```python
from build123d import *

# Parameters (mm, degrees)
SKETCH1_W                                    = 60
SKETCH1_H                                    = 60
BOSS_EXTRUDE1_DEPTH                          = 3
SKETCH2_R                                    = 10.25
CUT_EXTRUDE1_DEPTH                           = 43.532340636
SKETCH3_R                                    = 1.45
SERVO_Y_MOUNT_D2P9_DEPTH                     = 3.01
SKETCH4_R                                    = 1.45
CUT_EXTRUDE5_DEPTH                           = 43.532340636
SKETCH5_R                                    = 1.2
GUIDERAIL1_D2P4_DEPTH                        = 3.01
SKETCH6_R                                    = 1.2
GUIDEBLOCK2_D2P4_DEPTH                       = 3.01
SKETCH7_R                                    = 2.1
GUIDEBLOCK2_HEADCOUNTERBORE_D4P2_DEPTH       = 2.05
SKETCH8_R                                    = 1.7
BENCH_XDROP_M3_CLEARANCE_HOLES_2X_D3P4_DEPTH = 3.5


with BuildPart() as part:
    # Sketch1 → Boss-Extrude1 (new body)
    with BuildSketch(Plane.XY):
        Rectangle(SKETCH1_W, SKETCH1_H)
    extrude(amount=BOSS_EXTRUDE1_DEPTH)

    # Sketch2 → Cut-Extrude1 (cut, through all)
    with BuildSketch(Plane.XY.offset(3)):
        Circle(SKETCH2_R)
    extrude(amount=-CUT_EXTRUDE1_DEPTH, mode=Mode.SUBTRACT)

    # Sketch3 → Servo_Y_Mount_D2p9 (cut)
    with BuildSketch(Plane(origin=(0, 0, 0), x_dir=(-1, 0, 0), z_dir=(0, 0, -1))):
        with Locations((18, -25)):
            Circle(SKETCH3_R)
        with Locations((25, -25)):
            Circle(SKETCH3_R)
    extrude(amount=-SERVO_Y_MOUNT_D2P9_DEPTH, mode=Mode.SUBTRACT)

    # Sketch4 → Cut-Extrude5 (cut, through all)
    with BuildSketch(Plane(origin=(0, 0, 0), x_dir=(-1, 0, 0), z_dir=(0, 0, -1))):
        with Locations((17, 27)):
            Circle(SKETCH4_R)
        with Locations((23, 27)):
            Circle(SKETCH4_R)
    extrude(amount=-CUT_EXTRUDE5_DEPTH, mode=Mode.SUBTRACT)

    # Sketch5 → GuideRail1_D2p4 (cut)
    with BuildSketch(Plane.XY.offset(3)):
        with Locations((-24, -15)):
            Circle(SKETCH5_R)
        with Locations((-24, 0)):
            Circle(SKETCH5_R)
        with Locations((-24, 15)):
            Circle(SKETCH5_R)
    extrude(amount=-GUIDERAIL1_D2P4_DEPTH, mode=Mode.SUBTRACT)

    # Sketch6 → GuideBlock2_D2p4 (cut)
    with BuildSketch(Plane.XY.offset(3)):
        with Locations((0, -28)):
            Circle(SKETCH6_R)
        with Locations((0, -20)):
            Circle(SKETCH6_R)
    extrude(amount=-GUIDEBLOCK2_D2P4_DEPTH, mode=Mode.SUBTRACT)

    # Sketch7 → GuideBlock2_HeadCounterbore_D4p2 (cut)
    with BuildSketch(Plane.XY.offset(3)):
        with Locations((0, -28)):
            Circle(SKETCH7_R)
        with Locations((0, -20)):
            Circle(SKETCH7_R)
    extrude(amount=-GUIDEBLOCK2_HEADCOUNTERBORE_D4P2_DEPTH, mode=Mode.SUBTRACT)

    # Sketch8 → Bench_XDrop_M3_Clearance_Holes_2x_D3p4 (cut)
    with BuildSketch(Plane.XY.offset(3)):
        with Locations((-27, 28)):
            Circle(SKETCH8_R)
        with Locations((-13, 28)):
            Circle(SKETCH8_R)
    extrude(amount=-BENCH_XDROP_M3_CLEARANCE_HOLES_2X_D3P4_DEPTH, mode=Mode.SUBTRACT)


solid = part.part
```
Work out the finished part from the listing and answer in its coordinate system (mm). A direction names the side the tool comes from. Coordinates: 2 decimals unless noted, no trailing zeros. Loops run counter-clockwise (first coordinate to the right, second up) from the corner with the lowest first, then second, coordinate; pieces in that order, holes last.
1) For faces 4 (the flat face through (13, 0, 3)), 5 (the cylindrical face through (0.08, -25.9, 1.99)), determine the directions among +Z, -Z, +X, -X, +Y, -Y from which every point of the face is accessible in a straight line to the end or side of a thin tool.
Results:
face 4: +Z, +X, -X, +Y, -Y
face 5: +Z
2) Consider probe 1 along Y at (x, z) = (0, 0.65); probe 2 along Y at (x, z) = (0, 2.5); probe 3 along Y at (x, z) = (-24, 2.05). Determine where each line is inside the solid, lowest interval first.
Results:
probe 1: y = -30 to -29.2, -26.8 to -21.2, -18.8 to -10.25, 10.25 to 30
probe 2: y = -25.9 to -22.1, -17.9 to -10.25, 10.25 to 30
probe 3: y = -30 to -26.05, -23.95 to -16.2, -13.8 to -1.2, 1.2 to 13.8, 16.2 to 25.95, 28.05 to 30
3) For a pull along X with two mould halves and no side action, classify faces 1 (the cylindrical face through (-24.26, 13.83, 1.52)), 2 (the flat face through (-0.4, -30, 0.8)), 3 (the flat face through (-30, 0, 1)) as +X half, -X half, draft (parallel to the pull), parting line (faces both ways), or undercut.
Results:
face 1: undercut
face 2: draft
face 3: -X half
4) Section B-B (x = -6) is taken. Give the vertices of the cut face in (y, z), plus the area to 3 significant figures.
Results:
outline: (-30, 0) - (-8.31, 0) - (-8.31, 3) - (-30, 3) - close; (8.31, 0) - (30, 0) - (30, 3) - (8.31, 3) - close
area: 130 mm2
5) Section A-A (y = -28) is taken. Give the vertices of the cut face in (x, z), plus the area to 3 significant figures.
Results:
outline: (-30, 0) - (-1.2, 0) - (-1.2, 0.95) - (-2.1, 0.95) - (-2.1, 3) - (-30, 3) - close; (1.2, 0) - (30, 0) - (30, 3) - (2.1, 3) - (2.1, 0.95) - (1.2, 0.95) - close
area: 169 mm2
6) Section C-C (y = 15) is taken. Give the vertices of the cut face in (x, z), plus the area to 3 significant figures.
Results:
outline: (-30, 0) - (-25.2, 0) - (-25.2, 3) - (-30, 3) - close; (-22.8, 0) - (30, 0) - (30, 3) - (-22.8, 3) - close
area: 173 mm2
7) Section D-D (z = 1.7) is taken. Give the number of separate pieces and of enclosed holes in the cut face, plus the area to 3 significant figures.
Results:
separate pieces: 1
enclosed holes: 11
area: 3,180 mm2
8) A flat-ended cylindrical pin translates along its axis: pin 1 (4 mm diameter, centred on x = 0, y = -20, fed in from +Z). Find the tip coordinate at first contact, or state that the pin passes through.
Results:
pin 1: stops at z = 0.95
